```python
from build123d import *

# Parameters (mm, degrees)
BOSS_EXTRUDE1_DEPTH = 14
SKETCH3_OUTSIDE_W   = 44.278
SKETCH3_OUTSIDE_H   = 44.278
SKETCH3_OUTSIDE_R   = 3
CUT_EXTRUDE1_DEPTH  = 10


with BuildPart() as part:
    # Sketch1 → Revolve1 (revolve)
    with BuildSketch(Plane(origin=(0, 0, 0), x_dir=(1, 0, 0), z_dir=(0, 1, 0))):
        Polygon((0, 0), (0, 82.5), (11, 82.5), (11, 75.5), (5.865, 75.5), (5.865, 74), (4.365, 72.5), (4.365, 39.8), (6.25, 37.915), (6.25, 1.5), (4.75, 0), align=None)
    revolve(axis=Axis((0, 0, 0), (0, 0, -1)))

    # Sketch2 → Boss-Extrude1 (add)
    with BuildSketch(Plane.XY):
        Polygon((3.464101615, 0), (1.732050808, 3), (-1.732050808, 3), (-3.464101615, 0), (-1.732050808, -3), (1.732050808, -3), align=None)
    extrude(amount=BOSS_EXTRUDE1_DEPTH)

    # Sketch3 outside → Cut-Extrude1 (cut)
    with BuildSketch(Plane.XY.offset(14)):
        Rectangle(SKETCH3_OUTSIDE_W, SKETCH3_OUTSIDE_H)
        Circle(SKETCH3_OUTSIDE_R, mode=Mode.SUBTRACT)
    extrude(amount=-CUT_EXTRUDE1_DEPTH, mode=Mode.SUBTRACT)

    # Sketch4 → Cut-Revolve1 (revolve, cut)
    with BuildSketch(Plane(origin=(0, 0, 0), x_dir=(1, 0, 0), z_dir=(0, 1, 0))):
        with BuildLine():
            Line((3.464101615, -3), (3.464101615, -4))
            Line((3.464101615, -4), (3, -4))
            ThreePointArc((3, -4), (3.121679054, -3.448776291), (3.464101615, -3))
        make_face()
    revolve(axis=Axis((0, 0, 0), (0, 0, 1)), mode=Mode.SUBTRACT)


solid = part.part
```
Build history of the part. All positions in model axes, mm. A direction names the side the tool comes from. Give positions to 0.01 mm unless a question says otherwise; leave off trailing zeros. Loops run counter-clockwise (first coordinate to the right, second up) from the corner with the lowest first, then second, coordinate; pieces in that order, holes last.
Item 1: Drill centre lines: line 1 (Z direction, x = 3, y = -9.25); line 2 (X direction, y = -0.25, z = -35) (3 decimals); line 3 (X direction, y = -3.5, z = -47). Where is each one in solid material? Low to high.
Answers follow:
line 1: z = -82.5 to -75.5
line 2: x = -6.245 to 6.245
line 3: x = -2.61 to 2.61
Item 2: Pull direction Z, two halves, no side cores. Call faces 1 (the face through (3.1, 1, 0)), 2 (the face through (-4.654, 3.569, -74.74)), 3 (the face through (0, -3, 2)): released by +Z, released by -Z, zero draft, split by the parting line, or undercut.
Answers follow:
face 1: released by +Z
face 2: undercut
face 3: zero draft
Item 3: Flat gauge pins, fed straight in: pin 1 (1 mm diameter, centred on x = 0, z = 3, fed in from -Y); pin 2 (10 mm diameter, centred on y = -8.5, z = -28, fed in from +X); pin 3 (1.5 mm diameter, centred on x = -5, y = -3, fed in from +Z). Where does each tip first touch, or does it go through?
Answers follow:
pin 1: stops at y = -3
pin 2: stops at x = 5.18
pin 3: stops at z = -0.33
Item 4: Slice it at A-A, the plane z = -15. List the corners of the cut face in (x, y).
Answers follow:
outline: circle Ø12.5 at (0, 0)
Item 5: Which spindle directions (+Z, -Z, +X, -X, +Y, -Y) get a long thin tool onto all of the face, cutting with end or side? Do faces 4 (the face through (-3.217, -2.95, -55.921)), 5 (the face through (0, 3, 2)), 6 (the face through (-2.6, 1.5, 1.5)), 7 (the face through (-3, 0, 9)). Say none if no direction does.
Answers follow:
face 4: none
face 5: +Z, +X, -X, +Y
face 6: +Z, -X, +Y
face 7: +Z
